from build123d import *

# Parameters (mm, degrees)
SKETCH2_R           = 32.258
SKETCH2_R_2         = 27.305
BOSS_EXTRUDE1_DEPTH = 4.7625
SKETCH3_R           = 1.651
CUT_EXTRUDE1_DEPTH  = 5.7625
CIRPATTERN1_COUNT   = 4


with BuildPart() as part:
    # Sketch2 → Boss-Extrude1 (new body)
    with BuildSketch(Plane(origin=(0, 0, 0), x_dir=(1, 0, 0), z_dir=(0, 1, 0))):
        Circle(SKETCH2_R)
        Circle(SKETCH2_R_2, mode=Mode.SUBTRACT)
    extrude(amount=BOSS_EXTRUDE1_DEPTH)

    # Sketch3 → Cut-Extrude1 (cut, through all)
    with BuildSketch(Plane(origin=(0, 4.7625, 0), x_dir=(1, 0, 0), z_dir=(0, 1, 0))):
        with Locations((0, 29.7815)):
            Circle(SKETCH3_R)
    cut_extrude1 = extrude(amount=-CUT_EXTRUDE1_DEPTH, mode=Mode.SUBTRACT)

    # CirPattern1: Cut-Extrude1 ×4 about axis
    cirpattern1_axis = Axis((0, 0, 0), (0, 1, 0))
    for i in range(1, CIRPATTERN1_COUNT):
        add(cut_extrude1.rotate(cirpattern1_axis, i * 360 / CIRPATTERN1_COUNT), mode=Mode.SUBTRACT)


solid = part.part
Source: CAD feature listing. Evaluate the final solid. Frame: model axes, mm. Round coordinates to 2 decimals unless told otherwise and drop trailing zeros. Loops run counter-clockwise (first coordinate to the right, second up) from the corner with the lowest first, then second, coordinate; pieces in that order, holes last. Notation, with made-up numbers: M 1,37.5 L 32,37.5 A20 ccw 32,49.5 Z; hole C 40.5,-7.75 d3. An arc over 180 degrees is marked long. Answer as CSV lines item,"result".
Q1. Cut plane A-A (z = 0). Return the cut outline in (x, y) (1 decimal).
Verdict:
outline,"M -32.3,0 L -31.4,0 L -31.4,4.8 L -32.3,4.8 Z; M -28.1,0 L -27.3,0 L -27.3,4.8 L -28.1,4.8 Z; M 27.3,0 L 28.1,0 L 28.1,4.8 L 27.3,4.8 Z; M 31.4,0 L 32.3,0 L 32.3,4.8 L 31.4,4.8 Z"
Q2. Cut plane C-C (z = 7.5). Return the cut outline in (x, y).
Verdict:
outline,"M -31.37,0 L -26.25,0 L -26.25,4.76 L -31.37,4.76 Z; M 26.25,0 L 31.37,0 L 31.37,4.76 L 26.25,4.76 Z"
Q3. Cut plane B-B (x = 0). Return the cut outline in (y, z) (1 decimal).
Verdict:
outline,"M 0,-32.3 L 4.8,-32.3 L 4.8,-31.4 L 0,-31.4 Z; M 0,-28.1 L 4.8,-28.1 L 4.8,-27.3 L 0,-27.3 Z; M 0,27.3 L 4.8,27.3 L 4.8,28.1 L 0,28.1 Z; M 0,31.4 L 4.8,31.4 L 4.8,32.3 L 0,32.3 Z"
Q4. Line query: line 1 along Z through (x, y) = (0, 2.75) (1 decimal); line 2 along X through (y, z) = (2.1, 29). Output: solid intervals per line, ascending.
Verdict:
line 1,"z = -32.3 to -31.4, -28.1 to -27.3, 27.3 to 28.1, 31.4 to 32.3"
line 2,"x = -14.13 to -1.45, 1.45 to 14.13"
Q5. Cut plane D-D (x = -12.5). Return the cut outline in (y, z), plus the area to 3 significant figures.
Verdict:
outline,"M 0,-29.74 L 4.76,-29.74 L 4.76,-24.28 L 0,-24.28 Z; M 0,24.28 L 4.76,24.28 L 4.76,29.74 L 0,29.74 Z"
area,"52.0 mm^2"
Q6. Pull-direction query (X, two-part tool) for faces 1 (the face through (-17, 4.762, -22)), 2 (the face through (30.77, 2.35, -9.69)), 3 (the face through (0.89, 2.41, -31.17)); classes: +X half, -X half, draft (parallel to the pull), parting line (faces both ways), or undercut.
Verdict:
face 1,"draft"
face 2,"parting line"
face 3,"undercut"
Q7. Contact query for flat-ended pins moving along their axis: pin 1 (2 mm diameter, centred on x = -24, y = 2.5, fed in from +Z); pin 2 (2 mm diameter, centred on y = 4, z = 6.5, fed in from -X). Output: stop coordinate, or through.
Verdict:
pin 1,"stops at z = 22.62"
pin 2,"stops at x = -31.79"
